Check sheet for the drawn part. Datum: minimum x, y, z corner. Units: mm. A direction names the side the tool comes from. Round coordinates to 2 decimals unless told otherwise and drop trailing zeros. Write each loop counter-clockwise with the first axis right and the second up, starting at its lowest first coordinate (ties: lowest second). Pieces come first, ordered by that corner, then holes.
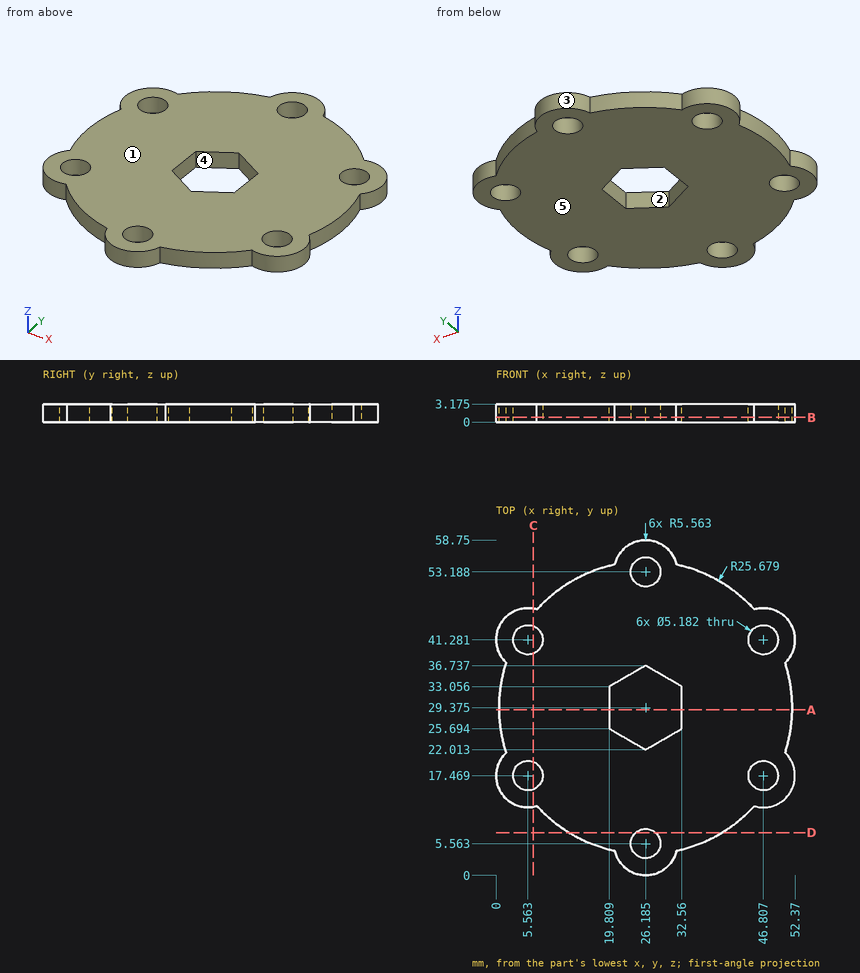
1. Release check for a two-part mould opening along X. For the marked faces 3, 4 and 5 record: released by +X, released by -X, zero draft, split by the parting line, or undercut.
2. Sectioned sample at A-A, the plane y = 29. Enter the section's corners in (x, z) (1 decimal).
3. Scan lines: line 1 along Y through (x, z) = (47, 0.65) (1 decimal); line 2 along Y through (x, z) = (26, 0.4) (1 decimal); line 3 along Y through (x, z) = (28, 0.55) (1 decimal). Record each from-to range of solid material in increasing order.
4. Sectioned sample at B-B, the plane z = 0.85. Give the number of separate pieces and of enclosed holes in the cut face, plus the area to 3 significant figures.
5. Sectioned sample at C-C, the plane x = 6.5. Enter the section's corners in (y, z) (1 decimal).
6. Set-up check for the marked faces 1 and 2: record each of +Z, -Z, +X, -X, +Y, -Y from which the full face is reachable in a straight line by a thin tool's end or side.
7. Go/stop test with flat-tipped pins: pin 1 (3 mm diameter, centred on x = 26.18, y = 5.56, fed in from -Z); pin 2 (1.5 mm diameter, centred on x = 23.5, z = 1.5, fed in from +Y). Record where each tip stops, or that it passes through.
8. Sectioned sample at D-D, the plane y = 7.5. Enter the section's corners in (x, z) (1 decimal).
Computed values:
1. face 3: split by the parting line
1. face 4: undercut
1. face 5: zero draft
2. outline: (0.5, 0) - (19.8, 0) - (19.8, 3.2) - (0.5, 3.2) - close; (32.6, 0) - (51.9, 0) - (51.9, 3.2) - (32.6, 3.2) - close
3. line 1: y = 11.9 to 14.9, 20.1 to 38.7, 43.9 to 46.8
3. line 2: y = 0 to 3, 8.1 to 22.1, 36.6 to 50.6, 55.8 to 58.7
3. line 3: y = 0.3 to 3.7, 7.4 to 23.1, 35.7 to 51.3, 55 to 58.4
4. separate pieces: 1
4. enclosed holes: 7
4. area: 1,990 mm2
5. outline: (12, 0) - (15.1, 0) - (15.1, 3.2) - (12, 3.2) - close; (19.9, 0) - (38.9, 0) - (38.9, 3.2) - (19.9, 3.2) - close; (43.7, 0) - (46.8, 0) - (46.8, 3.2) - (43.7, 3.2) - close
6. face 1: +Z, +X, -X, +Y, -Y
6. face 2: +Z, -Z
7. pin 1: passes through
7. pin 2: stops at y = 58.4
8. outline: (12.7, 0) - (24.5, 0) - (24.5, 3.2) - (12.7, 3.2) - close; (27.9, 0) - (39.6, 0) - (39.6, 3.2) - (27.9, 3.2) - close
